Geometry check sheet. Reference: the model listing, model coordinates, mm. A direction names the side the tool comes from. Round coordinates to 2 decimals unless told otherwise and drop trailing zeros. Order: outer loops, then holes, each group sorted by start corner. A loop starts at its lowest first (then second) coordinate and runs counter-clockwise, first axis right, second up. Notation, with made-up numbers: (50, 0) - (89, 0) arc R30 cw to (89, 30) - close; hole circle Ø1 at (74, -37). An arc over 180 degrees is marked (long way). Return JSON: item names as keys, results as strings. Group by question number.
Q1. Sectioned sample at C-C, the plane y = -5.25. Record the cut outline in (x, z), then the cut area to 3 significant figures.
Q2. Tool access check on faces 1 (the flat face through (-39, -23.525, 2)), 2 (the flat face through (-35.985, -13, -3)), 3 (the flat face through (-39, -13, -6.2)), 4 (the cylindrical face through (-1.203, 1.479, -1.141)), 5 (the flat face through (-23, 1, 0)). Record the directions out of +Z, -Z, +X, -X, +Y, -Y that give a thin tool (end or side, any length) a straight path to the whole face; none if there is none.
Q3. Gauge pin test, flat ends, axial feed: pin 1 Ø5 at (x, y) = (-39, -17.5) entering from +Z; pin 2 Ø7 at (x, y) = (-39.5, -12) entering from -Z; pin 3 Ø9.5 at (y, z) = (-13.5, -2) entering from +X. Record the tip position at first contact, or that the pin passes through.
Q4. Draft check along Z on faces 6 (the flat face through (-21, 1, -22.25)), 7 (the flat face through (-42.285, -9, -6)), 8 (the flat face through (-39, -25, 5.8)), 9 (the cylindrical face through (-6.907, 1.479, -11.587)). Enter one of: pulls with the +Z half, pulls with the -Z half, needs draft (parallel to the pull), parting line crosses it, or undercut.
Q5. Sectioned sample at D-D, the plane x = -23. Record the cut outline in (y, z).
Q6. Sectioned sample at A-A, the plane z = -10. Record the cut outline in (x, y).
Q7. Sectioned sample at B-B, the plane x = -5.69. Record the cut outline in (y, z).
Q8. Material ranges on line 1 along X through (y, z) = (1.35, -10); line 2 along Y through (x, z) = (-38.5, -6.75), recorded low to high.
```python
from build123d import *

# Parameters (mm, degrees)
SKETCH1_R           = 2
SKETCH1_W           = 6.3
SKETCH1_H           = 5
BOSS_EXTRUDE1_DEPTH = 3
SKETCH4_W           = 6.3
SKETCH4_H           = 5
BOSS_EXTRUDE3_DEPTH = 23.525
SKETCH5_W           = 6.3
SKETCH5_H           = 12
BOSS_EXTRUDE4_DEPTH = 2.75


with BuildPart() as part:
    # Sketch1 → Boss-Extrude1 (new body)
    # profile 1 of 2: a face of its own
    with BuildSketch(Plane(origin=(0, 0, 0), x_dir=(1, 0, 0), z_dir=(0, 1, 0))):
        with BuildLine():
            Line((-35.984691362, 0), (-4, 0))
            ThreePointArc((-4, 0), (-1.171572875, 1.171572875), (0, 4))
            Line((0, 4), (0, 20))
            Line((0, 20), (0, 22.25))
            Line((0, 22.25), (-42.284691362, 22.25))
            Line((-42.284691362, 22.25), (-42.284691362, 20))
            Line((-42.284691362, 20), (-42.284691362, 5))
            Line((-42.284691362, 5), (-35.984691362, 5))
            Line((-35.984691362, 5), (-35.984691362, 0))
        make_face()
        with Locations(Location((-5.69, 10, 0), (0, 0, 270))):
            Circle(SKETCH1_R, mode=Mode.SUBTRACT)
    # profile 2 of 2: a face of its own
    with BuildSketch(Plane(origin=(0, 0, 0), x_dir=(1, 0, 0), z_dir=(0, 1, 0))):
        with Locations((-39.134691362, 2.5)):
            Rectangle(SKETCH1_W, SKETCH1_H)
    extrude(amount=BOSS_EXTRUDE1_DEPTH)

    # Sketch4 → Boss-Extrude3 (add)
    with BuildSketch(Plane.XZ):
        with Locations((-39.134691362, -3.7)):
            Rectangle(SKETCH4_W, SKETCH4_H)
    extrude(amount=BOSS_EXTRUDE3_DEPTH)

    # Sketch5 → Boss-Extrude4 (add)
    with BuildSketch(Plane(origin=(0, -23.525, 0), x_dir=(-1, 0, 0), z_dir=(0, -1, 0))):
        with Locations((39.134691362, 0.2)):
            Rectangle(SKETCH5_W, SKETCH5_H)
    extrude(amount=BOSS_EXTRUDE4_DEPTH)


solid = part.part
```
Reply:
{
 "1": {"outline": "(-42.28, -6.2) - (-35.98, -6.2) - (-35.98, -1.2) - (-42.28, -1.2) - close", "area": "31.5 mm^2"},
 "2": {"face 1": "+Z, +X, -X", "face 2": "+Z, -Z, +X, -Y", "face 3": "-Z, +X, -X, -Y", "face 4": "+Z, +X, +Y, -Y", "face 5": "+Z, +X, -X, +Y"},
 "3": {"pin 1": "z = -1.2", "pin 2": "z = -6.2", "pin 3": "x = -35.98"},
 "4": {"face 6": "pulls with the -Z half", "face 7": "needs draft", "face 8": "pulls with the +Z half", "face 9": "undercut"},
 "5": {"outline": "(0, -22.25) - (3, -22.25) - (3, 0) - (0, 0) - close"},
 "6": {"outline": "(-42.28, 0) - (-7.69, 0) - (-7.69, 3) - (-42.28, 3) - close; (-3.69, 0) - (0, 0) - (0, 3) - (-3.69, 3) - close"},
 "7": {"outline": "(0, -22.25) - (3, -22.25) - (3, -12) - (0, -12) - close; (0, -8) - (3, -8) - (3, 0) - (0, 0) - close"},
 "8": {"line 1": "-42.28 to -7.69, -3.69 to 0", "line 2": "0 to 3"}
}
